```python
from build123d import *

# Parameters (mm, degrees)
F1_W     = 200
F1_H     = 240
F2_DEPTH = 20
F3_R     = 6.35
F4_DEPTH = 30
F5_SIZE  = 2
F6_R     = 10
F7_R     = 12.7
F8_DEPTH = 10


with BuildPart() as f2:
    # F1 (on Front) → F2 (new body)
    with BuildSketch(Plane.XZ):
        with Locations((0, 40)):
            Rectangle(F1_W, F1_H)
    extrude(amount=-F2_DEPTH)

    # F3 (on Front) → F4 (join)
    with BuildSketch(Plane.XZ):
        with Locations((0, 92)):
            Circle(F3_R)
        Circle(F3_R)
    extrude(amount=F4_DEPTH)

    # F5
    f5_edges = [f2.edges().sort_by_distance(p)[0] for p in [
        (-6.35, -30, 92),
        (-6.35, -30, 0),
    ]]
    chamfer(f5_edges, length=F5_SIZE)

    # F6
    f6_edges = [f2.edges().sort_by_distance(p)[0] for p in [
        (-100, 10, 160),
        (-100, 10, -80),
        (100, 10, -80),
        (100, 10, 160),
    ]]
    fillet(f6_edges, radius=F6_R)

    # F7 (on face) → F8 (join)
    with BuildSketch(Plane.XZ):
        Circle(F7_R)
    extrude(amount=F8_DEPTH)


solid = f2.part
```
Input: part model. Units: mm. Frame: model coordinates. A direction names the side the tool comes from. Give positions to 0.01 mm unless a question says otherwise; leave off trailing zeros. Order: outer loops, then holes, each group sorted by start corner. A loop starts at its lowest first (then second) coordinate and runs counter-clockwise, first axis right, second up.
1. Cut plane A-A (z = 92). Return loops of the section in (x, y), and give its area (3 significant figures).
Computed:
outline: (-100, 0) - (-6.35, 0) - (-6.35, -28) - (-4.35, -30) - (4.35, -30) - (6.35, -28) - (6.35, 0) - (100, 0) - (100, 20) - (-100, 20) - close
area: 4,380 mm2
2. Cut plane D-D (x = -24.5). Return loops of the section in (y, z), and give its area (3 significant figures).
Computed:
outline: (0, -80) - (20, -80) - (20, 160) - (0, 160) - close
area: 4,800 mm2
3. Cut plane C-C (z = 0). Return loops of the section in (x, y), and give its area (3 significant figures).
Computed:
outline: (-100, 0) - (-12.7, 0) - (-12.7, -10) - (-6.35, -10) - (-6.35, -28) - (-4.35, -30) - (4.35, -30) - (6.35, -28) - (6.35, -10) - (12.7, -10) - (12.7, 0) - (100, 0) - (100, 20) - (-100, 20) - close
area: 4,500 mm2
4. Pin query (flat end, axial travel): pin 1 Ø4 at (x, z) = (38, 94) entering from -Y; pin 2 Ø4 at (y, z) = (-4.5, 92) entering from +X. Return the tip coordinate at first contact, or that it passes through.
Computed:
pin 1: stops at y = 0
pin 2: stops at x = 6.35
5. Draft query along Z for faces 3 (the face through (3, -10, 6)), 4 (the face through (-1, 10, 160)), 5 (the face through (100, 10, 38)). Return one class per face: released by +Z, released by -Z, zero draft, split by the parting line, or undercut.
Computed:
face 3: undercut
face 4: released by +Z
face 5: zero draft
6. Line query: probe 1 along Y at (x, z) = (-10.5, 128); probe 2 along X at (y, z) = (-17, -3). Output: solid intervals per line, ascending.
Computed:
probe 1: y = 0 to 20
probe 2: x = -5.6 to 5.6
7. Cut plane B-B (x = 0). Return loops of the section in (y, z), and give its area (3 significant figures).
Computed:
outline: (-30, -4.35) - (-28, -6.35) - (-10, -6.35) - (-10, -12.7) - (0, -12.7) - (0, -80) - (20, -80) - (20, 160) - (0, 160) - (0, 98.35) - (-28, 98.35) - (-30, 96.35) - (-30, 87.65) - (-28, 85.65) - (0, 85.65) - (0, 12.7) - (-10, 12.7) - (-10, 6.35) - (-28, 6.35) - (-30, 4.35) - close
area: 5,680 mm2
8. Set-up query: faces 1 (the face through (0, -30, 0)), 2 (the face through (-1.38, -13.8, 85.8)). Return all of +Z, -Z, +X, -X, +Y, -Y with unobstructed straight access to the full face (end or side cutting, diameter ignored); none if empty.
Computed:
face 1: +Z, -Z, +X, -X, -Y
face 2: -Y
